Source: CAD feature listing. Evaluate the final solid. Frame: model axes, mm. Give positions to 0.01 mm unless a question says otherwise; leave off trailing zeros. Order: outer loops, then holes, each group sorted by start corner. A loop starts at its lowest first (then second) coordinate and runs counter-clockwise, first axis right, second up. Notation, with made-up numbers: M 81,61 L 100,61 A19 cw 100,95 Z; hole C 84,33.25 d6. An arc over 180 degrees is marked long. Use CSV: the item, a comma, the result in double quotes. Start each with the question number.
Item 1: Section query A-A on y = 9.8. Count the separate pieces of the cut face and the enclosed holes in it, and give its area (3 significant figures).
Item 2: Section query B-B on z = -463. Return loops of the section in (x, y).
Item 3: Ray query, probe 1 along X at (y, z) = (10.45, -226.5); probe 2 along X at (y, z) = (10.1, -330); probe 3 along X at (y, z) = (8.95, 422). Return the intervals inside material, ascending. Write a range as from..to.
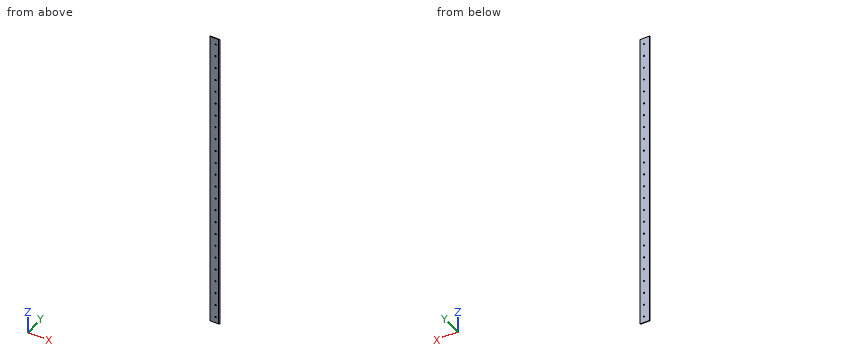
from build123d import *

# Parameters (mm, degrees)
BOSS_EXTRUDE3_DEPTH    = 609.6
F_10_CLEARANCE_HOLE3_D = 5.1054
LPATTERN1_COUNT        = 24
LPATTERN1_PITCH        = 50.8


with BuildPart() as part:
    # Sketch1<4> → Boss-Extrude3 (new, symmetric)
    with BuildSketch(Plane.XY):
        with BuildLine():
            ThreePointArc((-4.443185344, 8.636), (-2.498384078, 10.316985791), (0, 10.922))
            Line((0, 10.922), (-38.1, 10.922))
            Line((-38.1, 10.922), (-38.1, 8.636))
            Line((-38.1, 8.636), (-4.443185344, 8.636))
        make_face()
    extrude(amount=BOSS_EXTRUDE3_DEPTH, both=True)

    # #10 Clearance Hole3 (through all)
    with Locations(Plane(origin=(0, 10.922, 0), x_dir=(1, 0, 0), z_dir=(0, 1, 0))):
        with Locations((-15.875, -584.2)):
            f_10_clearance_hole3 = Hole(F_10_CLEARANCE_HOLE3_D / 2)

    # LPattern1: #10 Clearance Hole3 ×24
    with Locations(*[(0, 0, -i * LPATTERN1_PITCH) for i in range(1, LPATTERN1_COUNT)]):
        add(f_10_clearance_hole3, mode=Mode.SUBTRACT)


solid = part.part
Verdict:
1,separate pieces,"1"
1,enclosed holes,"24"
1,area,"41,900 mm2"
2,outline,"M -38.1,8.64 L -4.44,8.64 A5.46 cw 0,10.92 L -38.1,10.92 Z"
3,probe 1,"-38.1..-17.33, -14.42..-2.22"
3,probe 2,"-38.1..-18.42, -13.33..-2.88"
3,probe 3,"-38.1..-4.2"
